```python
from build123d import *

# Parameters (mm, degrees)
SKETCH_1_W          = 48
SKETCH_1_H          = 17
EXTRUDE_1_DEPTH     = 1
SKETCH_2_W          = 29
SKETCH_2_H          = 17
EXTRUDE_2_DEPTH     = 4
SKETCH_3_W          = 27
SKETCH_3_H          = 16
CUT_EXTRUDE_1_DEPTH = 4
SKETCH_4_W          = 22
SKETCH_4_H          = 11.5
CUT_EXTRUDE_2_DEPTH = 6
CHAMFER_1_SIZE      = 1.5
SKETCH_5_R          = 0.5
CUT_EXTRUDE_3_DEPTH = 2
SKETCH_6_W          = 9.5
SKETCH_6_H          = 1
CUT_EXTRUDE_4_DEPTH = 0.5


with BuildPart() as part:
    # 草图1 → 凸台-拉伸1 (new body)
    with BuildSketch(Plane(origin=(0, 0, 0), x_dir=(1, 0, 0), z_dir=(0, 1, 0))):
        Rectangle(SKETCH_1_W, SKETCH_1_H)
    extrude(amount=EXTRUDE_1_DEPTH)

    # 草图2 → 凸台-拉伸2 (add)
    with BuildSketch(Plane(origin=(0, 1, 0), x_dir=(1, 0, 0), z_dir=(0, 1, 0))):
        Rectangle(SKETCH_2_W, SKETCH_2_H)
    extrude(amount=EXTRUDE_2_DEPTH)

    # 草图3 → 切除-拉伸1 (cut)
    with BuildSketch(Plane.XZ):
        with Locations((0, 0.5)):
            Rectangle(SKETCH_3_W, SKETCH_3_H)
    extrude(amount=-CUT_EXTRUDE_1_DEPTH, mode=Mode.SUBTRACT)

    # 草图4 → 切除-拉伸2 (cut, through all)
    with BuildSketch(Plane(origin=(0, 5, 0), x_dir=(1, 0, 0), z_dir=(0, 1, 0))):
        with Locations((0, -0.25)):
            Rectangle(SKETCH_4_W, SKETCH_4_H)
    extrude(amount=-CUT_EXTRUDE_2_DEPTH, mode=Mode.SUBTRACT)

    # 倒角1
    chamfer_1_edges = [part.edges().sort_by_distance(p)[0] for p in [
        (0, 5, -8.5),
    ]]
    chamfer(chamfer_1_edges, length=CHAMFER_1_SIZE)

    # 草图5 → 切除-拉伸3 (cut, through all)
    with BuildSketch(Plane(origin=(0, 1, 0), x_dir=(1, 0, 0), z_dir=(0, 1, 0))):
        with Locations((-22.5, 7)):
            Circle(SKETCH_5_R)
        with Locations((22.5, 7)):
            Circle(SKETCH_5_R)
        with Locations((22.5, -7)):
            Circle(SKETCH_5_R)
        with Locations((-22.5, -7)):
            Circle(SKETCH_5_R)
    extrude(amount=-CUT_EXTRUDE_3_DEPTH, mode=Mode.SUBTRACT)

    # 草图6 → 切除-拉伸4 (cut)
    with BuildSketch(Plane(origin=(0, 1, 0), x_dir=(1, 0, 0), z_dir=(0, 1, 0))):
        with Locations((-19.25, 4)):
            Rectangle(SKETCH_6_W, SKETCH_6_H)
        with Locations((-19.25, -4)):
            Rectangle(SKETCH_6_W, SKETCH_6_H)
        with Locations((19.25, -4)):
            Rectangle(SKETCH_6_W, SKETCH_6_H)
        with Locations((19.25, 4)):
            Rectangle(SKETCH_6_W, SKETCH_6_H)
    extrude(amount=-CUT_EXTRUDE_4_DEPTH, mode=Mode.SUBTRACT)


solid = part.part
```
Build history of the part. All positions in model axes, mm. A direction names the side the tool comes from. Round coordinates to 2 decimals unless told otherwise and drop trailing zeros. Loops run counter-clockwise (first coordinate to the right, second up) from the corner with the lowest first, then second, coordinate; pieces in that order, holes last.
Item 1: Which spindle directions (+Z, -Z, +X, -X, +Y, -Y) get a long thin tool onto all of the face, cutting with end or side? Do faces 1 (the face through (-19, 1, 6)), 2 (the face through (-13.5, 2, 0)), 3 (the face through (-19, 0.5, -4)). Say none if no direction does.
Item 2: Two-plate mould, pull along X, no slides. Class faces 4 (the face through (-24, 0.5, 0.1)), 5 (the face through (13.5, 2, 0)), 6 (the face through (-0.2, 4.5, 6)), 7 (the face through (0, 4, -8)): released by +X, released by -X, zero draft, split by the parting line, or undercut.
Item 3: Saw through at D-D (z = -4). List the corners of the cut face in (x, y).
Item 4: Drill centre lines: line 1 along X through (y, z) = (0.45, -7); line 2 along Z through (x, y) = (-22.5, 0.3); line 3 along X through (y, z) = (4.85, -3). Where is each one in solid material? Low to high.
Item 5: Saw through at C-C (x = -1). List the corners of the cut face in (y, z), then the cut area to 4 significant figures.
Item 6: Pin check, flat tips, straight feed: P1, Ø10, axis at x = -5, z = 4, coming from the +Y side; P2, Ø1.1, axis at y = 4.5, z = -1, coming from the -X side; P3, Ø5, axis at x = 4, z = -4.5, coming from the -Y side; P4, Ø1.1, axis at x = 17.5, z = 4, coming from the +Y side. Stop position of each tip, or through.
Item 7: Saw through at B-B (z = 7). List the corners of the cut face in (x, y), then the cut area to 3 significant figures.
Item 8: Saw through at A-A (x = -22.5). List the corners of the cut face in (y, z).
Worked answers:
1. face 1: +Z, -Z, -X, +Y
1. face 2: +Z, -Y
1. face 3: -X, +Y
2. face 4: released by -X
2. face 5: undercut
2. face 6: undercut
2. face 7: zero draft
3. outline: (-24, 0) - (-13.5, 0) - (-13.5, 4) - (-11, 4) - (-11, 5) - (-14.5, 5) - (-14.5, 0.5) - (-24, 0.5) - close; (11, 4) - (13.5, 4) - (13.5, 0) - (24, 0) - (24, 0.5) - (14.5, 0.5) - (14.5, 5) - (11, 5) - close
4. line 1: x = -24 to -23, -22 to -13.5, 13.5 to 22, 23 to 24
4. line 2: z = -8.5 to -7.5, -6.5 to 6.5, 7.5 to 8.5
4. line 3: x = -14.5 to -11, 11 to 14.5
5. outline: (0, -8.5) - (3.5, -8.5) - (5, -7) - (5, -5.5) - (4, -5.5) - (4, -7.5) - (0, -7.5) - close; (4, 6) - (5, 6) - (5, 8.5) - (4, 8.5) - close
5. area: 8.375 mm2
6. P1: stops at y = 5
6. P2: stops at x = -14.5
6. P3: stops at y = 4
6. P4: stops at y = 1
7. outline: (-24, 0) - (-23, 0) - (-23, 1) - (-24, 1) - close; (-22, 0) - (-13.5, 0) - (-13.5, 4) - (13.5, 4) - (13.5, 0) - (22, 0) - (22, 1) - (14.5, 1) - (14.5, 5) - (-14.5, 5) - (-14.5, 1) - (-22, 1) - close; (23, 0) - (24, 0) - (24, 1) - (23, 1) - close
7. area: 54.0 mm2
8. outline: (0, -8.5) - (1, -8.5) - (1, -7.5) - (0, -7.5) - close; (0, -6.5) - (1, -6.5) - (1, -4.5) - (0.5, -4.5) - (0.5, -3.5) - (1, -3.5) - (1, 3.5) - (0.5, 3.5) - (0.5, 4.5) - (1, 4.5) - (1, 6.5) - (0, 6.5) - close; (0, 7.5) - (1, 7.5) - (1, 8.5) - (0, 8.5) - close
